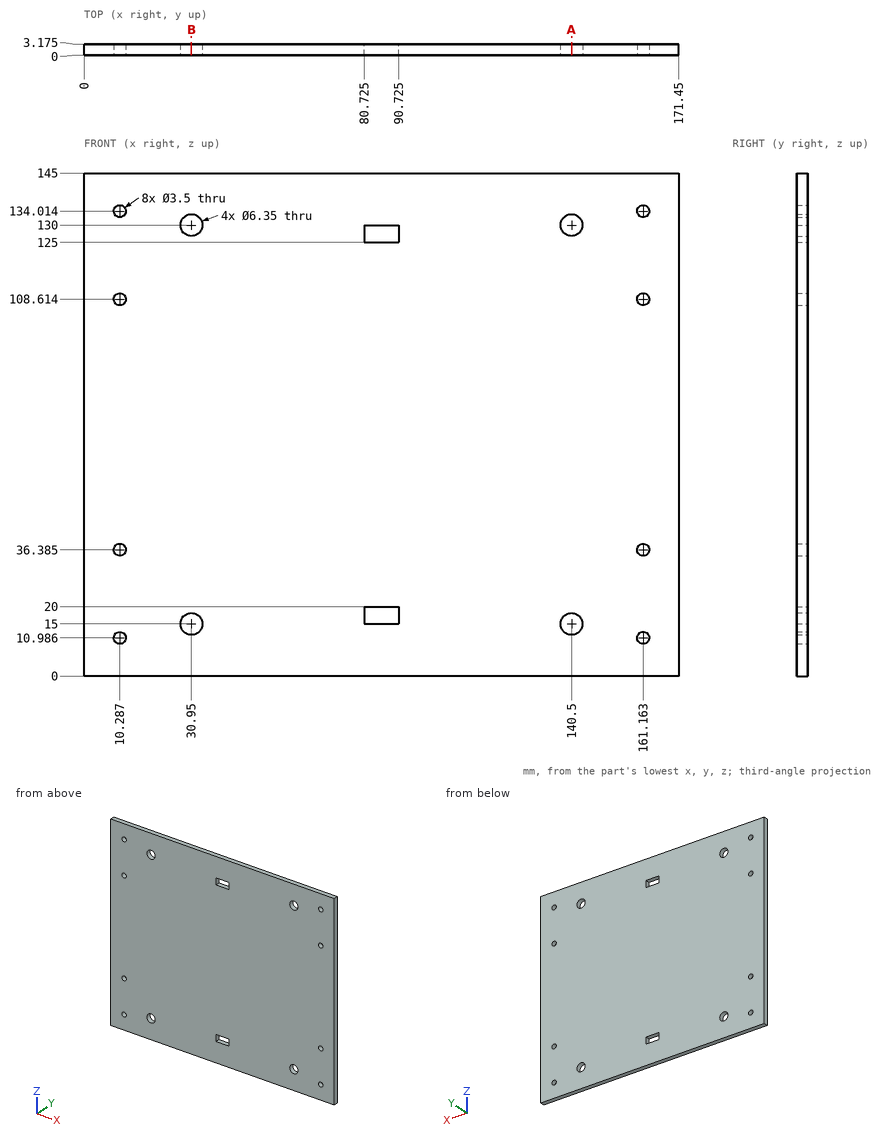
The drawing under review shows one solid part. Ordinate dimensions are in mm from its lowest x, y, z. Coordinates: 2 decimals unless noted, no trailing zeros. Loops run counter-clockwise (first coordinate to the right, second up) from the corner with the lowest first, then second, coordinate; pieces in that order, holes last.
Item 1: Wall thickness on L1, parallel to Z at x = 140.5, y = 1.55 (1 decimal); L2, parallel to X at y = 0.85, z = 36.5; L3, parallel to Z at x = 11.5, y = 2.45 (1 decimal): over which ranges is each line inside the solid? List them lowest first.
Completed:
L1: z = 0 to 11.8, 18.2 to 126.8, 133.2 to 145
L2: x = 0 to 8.54, 12.03 to 159.42, 162.91 to 171.45
L3: z = 0 to 9.7, 12.2 to 35.1, 37.6 to 107.4, 109.9 to 132.8, 135.3 to 145
Item 2: Add section A-A (x = 140.5). Write out the cut boundary in (y, z) (1 decimal).
Completed:
outline: (0, 0) - (3.2, 0) - (3.2, 11.8) - (0, 11.8) - close; (0, 18.2) - (3.2, 18.2) - (3.2, 126.8) - (0, 126.8) - close; (0, 133.2) - (3.2, 133.2) - (3.2, 145) - (0, 145) - close
Item 3: Clearance check with a flat-ended pin moving along its axis: pin 1 (3 mm diameter, centred on x = 10.29, z = 36.39, fed in from +Y). State where the tip first meets the part, or that it passes through.
Completed:
pin 1: passes through
